Work out the finished part from the listing and answer in its coordinate system (mm). A direction names the side the tool comes from. Give positions to 0.01 mm unless a question says otherwise; leave off trailing zeros. Order: outer loops, then holes, each group sorted by start corner. A loop starts at its lowest first (then second) coordinate and runs counter-clockwise, first axis right, second up. Notation, with made-up numbers: M 50.5,-14.5 L 67.5,-14.5 A28 cw 67.5,7.5 Z; hole C 37,5.25 d6. An arc over 180 degrees is marked long. One line per item, written item: value.
from build123d import *

# Parameters (mm, degrees)
CHAMFER1_SIZE      = 0.4
CUT_EXTRUDE1_START = -2.4000001
CUT_EXTRUDE1_DEPTH = 3.4000001
FILLET1_R          = 0.2


with BuildPart() as part:
    # Sketch1 → Revolve1 (revolve)
    with BuildSketch(Plane(origin=(0, 0, 0), x_dir=(0, 0, -1), z_dir=(1, 0, 0)), mode=Mode.PRIVATE) as revolve1_sk:
        with BuildLine():
            Line((30, 0), (30, 2.5))
            Line((30, 2.5), (0, 2.5))
            Line((0, 2.5), (0, 4.75))
            Line((0, 4.75), (-0.5, 4.75))
            ThreePointArc((-0.5, 4.75), (-2.374208166, 4.080480498), (-3.4, 2.375))
            Line((-3.4, 2.375), (-3.4, 0))
            Line((-3.4, 0), (30, 0))
        make_face()
    revolve(revolve1_sk.sketch.rotate(Axis((0, 0, 30.809969789), (0, 0, -1)), 90), axis=Axis((0, 0, 30.809969789), (0, 0, -1)))

    # Chamfer1
    chamfer1_edges = [part.edges().sort_by_distance(p)[0] for p in [
        (-2.5, 0, -30),
    ]]
    chamfer(chamfer1_edges, length=CHAMFER1_SIZE)

    # Sketch2 → Cut-Revolve1 (revolve, cut)
    with BuildSketch(Plane(origin=(0, 0, 0), x_dir=(0, 0, -1), z_dir=(1, 0, 0)), mode=Mode.PRIVATE) as cut_revolve1_sk:
        Polygon((-3.4, 0), (-3.4, 1.5), (-1, 1.5), (-0.133974596, 0), align=None)
    revolve(cut_revolve1_sk.sketch.rotate(Axis((0, 0, 2.452500839), (0, 0, -1)), 90), axis=Axis((0, 0, 2.452500839), (0, 0, -1)), mode=Mode.SUBTRACT)

    # Cut-Extrude1: read off the stored shape, not the designer's step
    # Cut-Extrude1 outline → Cut-Extrude1 (cut)
    with BuildSketch(Plane.XY.offset(3.4).offset(CUT_EXTRUDE1_START)):
        with BuildLine():
            Line((1.5, 0), (1.5, 0.866025404))
            Line((1.5, 0.866025404), (0.750000011, 1.299038099))
            ThreePointArc((0.750000011, 1.299038099), (1.299038109, 0.749999994), (1.5, 0))
        make_face()
        with BuildLine():
            ThreePointArc((-0.749999993, 1.29903811), (1e-08, 1.5), (0.750000011, 1.299038099))
            Line((0.750000011, 1.299038099), (0, 1.732050808))
            Line((0, 1.732050808), (-0.749999993, 1.29903811))
        make_face()
        with BuildLine():
            Line((1.5, -0.866025404), (1.5, 0))
            ThreePointArc((1.5, 0), (1.299038107, -0.749999997), (0.750000005, -1.299038103))
            Line((0.750000005, -1.299038103), (1.5, -0.866025404))
        make_face()
        with BuildLine():
            ThreePointArc((-1.5, 0), (-1.299038104, 0.750000003), (-0.749999993, 1.29903811))
            Line((-0.749999993, 1.29903811), (-1.5, 0.866025404))
            Line((-1.5, 0.866025404), (-1.5, 0))
        make_face()
        with BuildLine():
            Line((0, -1.732050808), (0.750000005, -1.299038103))
            ThreePointArc((0.750000005, -1.299038103), (3e-09, -1.5), (-0.75, -1.299038106))
            Line((-0.75, -1.299038106), (0, -1.732050808))
        make_face()
        with BuildLine():
            ThreePointArc((-0.75, -1.299038106), (-1.299038106, -0.75), (-1.5, 0))
            Line((-1.5, 0), (-1.5, -0.866025404))
            Line((-1.5, -0.866025404), (-0.75, -1.299038106))
        make_face()
    extrude(amount=CUT_EXTRUDE1_DEPTH, mode=Mode.SUBTRACT)

    # Cut-Extrude1 2 outline → Cut-Extrude1 2 (revolve)
    with BuildSketch(Plane.XZ):
        Polygon((1.732050837, 1.133974613), (1.499999957, 0.999999975), (1.732050808, 0.9999999), align=None)
    revolve(axis=Axis((0, 0, 0), (0, 0, 1)))

    # Fillet1
    fillet1_edges = [part.edges().sort_by_distance(p)[0] for p in [
        (-2.5, 0, 0),
    ]]
    fillet(fillet1_edges, radius=FILLET1_R)


solid = part.part
(1) Which of the six approach directions +Z, -Z, +X, -X, +Y, -Y give full straight-line access (tool end or side, diameter ignored) to faces 5 (the flat face through (-0.761, -1.293, 2.183)), 6 (the flat face through (-2.04, 2.04, 0)), 7 (the cylindrical face through (-1.03, 4.637, 0.254))?
Findings:
face 5: +Z
face 6: -Z
face 7: +Z, -Z
(2) Find the intervals of material crossed by probe 1 along Y at (x, z) = (2, -3); probe 2 along X at (y, z) = (2.25, 2), in increasing order. Write a range as from..to.
Findings:
probe 1: y = -1.5..1.5
probe 2: x = -3.71..3.71
(3) Section A-A, the plane z = -1 is taken. Give the vertices of the cut face in (x, y).
Findings:
outline: C 0,0 d5
(4) Determine the mould class of faces 1 (the flat face through (0, 0, -30)), 2 (the flat face through (1.5, 0, 2)), 3 (the flat face through (-1.5, 0, 2)), 4 (the cylindrical face through (-2.5, -0.1, -14.7)) for opening direction X: pulls with the +X half, pulls with the -X half, needs draft (parallel to the pull), parting line crosses it, or undercut.
Findings:
face 1: needs draft
face 2: undercut
face 3: undercut
face 4: parting line crosses it
(5) Given P1, Ø1.9, axis at y = 0, z = 2, coming from the +X side; P2, Ø0.9, axis at y = -0.5, z = 2.5, coming from the -X side; P3, Ø1.5, axis at x = 3, z = -12, coming from the +Y side, each flat-ended and moving along its own axis, determine where each tip first touches the part or whether it passes through.
Findings:
P1: stops at x = 4.7
P2: stops at x = -4.29
P3: stops at y = 1.09
